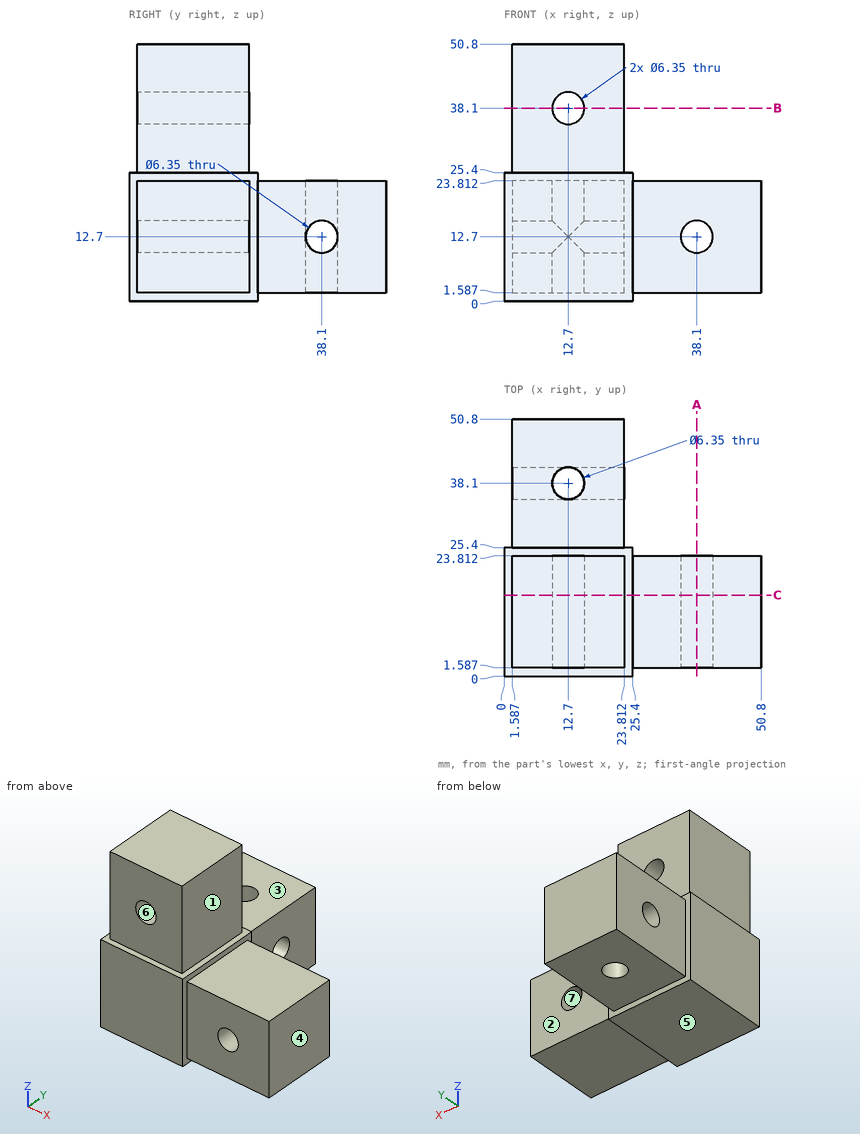
Source: three-view drawing plus pictorial views. Frame: mm from the lowest corner of the part. A direction names the side the tool comes from. Give positions to 0.01 mm unless a question says otherwise; leave off trailing zeros. Order: outer loops, then holes, each group sorted by start corner. A loop starts at its lowest first (then second) coordinate and runs counter-clockwise, first axis right, second up. Notation, with made-up numbers: (75, 72.25) -> (122, 72.25) arc R34 cw to (122, 108.25) -> close; hole circle Ø9 at (-10.5, -35). An arc over 180 degrees is marked (long way). Write each question's results on one line, items separated by ' | '. Start each with the question number.
Item 1: Cut plane B-B on z = 38.1. Return the cut outline in (x, y) (1 decimal).
Item 2: Contact query for flat-ended pins moving along their axis: P1, Ø11, axis at y = 40.5, z = 8, coming from the +X side; P2, Ø11, axis at x = 41.5, y = 14.5, coming from the +Z side; P3, Ø1.5, axis at x = 8, z = 40, coming from the +Y side. Output: stop coordinate, or through.
Item 3: Cut plane C-C on y = 16. Give the number of separate pieces and of enclosed holes in the cut face, then the cut area to 3 significant figures.
Item 4: Line query: line 1 (Z direction, x = 12.7, y = 13) (1 decimal); line 2 (X direction, y = 38.1, z = 18.5) (1 decimal). Output: solid intervals per line, ascending.
Item 5: Mould query, pull axis Z, two halves, no side actions, for the marked faces 4, 5, 6 and 7. Classes: pulls with the +Z half, pulls with the -Z half, needs draft (parallel to the pull), parting line crosses it, or undercut.
Item 6: Cut plane A-A on x = 38.1. Return the cut outline in (y, z) (1 decimal).
Item 7: Set-up query: the marked faces 1, 2 and 3. Return all of +Z, -Z, +X, -X, +Y, -Y with unobstructed straight access to the full face (end or side cutting, diameter ignored); none if empty.
Established:
1) outline: (1.6, 1.6) -> (9.5, 1.6) -> (9.5, 23.8) -> (1.6, 23.8) -> close; (15.9, 1.6) -> (23.8, 1.6) -> (23.8, 23.8) -> (15.9, 23.8) -> close
2) P1: x = 23.81 | P2: z = 23.81 | P3: y = 23.81
3) separate pieces: 1 | enclosed holes: 2 | area: 1,710 mm^2
4) line 1: 0 to 34.9, 41.3 to 50.8 | line 2: 1.6 to 9.5, 15.9 to 23.8
5) face 4: needs draft | face 5: pulls with the -Z half | face 6: undercut | face 7: undercut
6) outline: (1.6, 1.6) -> (23.8, 1.6) -> (23.8, 9.5) -> (1.6, 9.5) -> close; (1.6, 15.9) -> (23.8, 15.9) -> (23.8, 23.8) -> (1.6, 23.8) -> close
7) face 1: +Z, +X, +Y, -Y | face 2: +Z, -Z, +X, +Y | face 3: +Z, +X, -X, +Y
